Check sheet for the drawn part. Datum: minimum x, y, z corner. Units: mm. Give positions to 0.01 mm unless a question says otherwise; leave off trailing zeros. Write each loop counter-clockwise with the first axis right and the second up, starting at its lowest first coordinate (ties: lowest second). Pieces come first, ordered by that corner, then holes. Notation, with made-up numbers: M 25.5,80 L 47.5,80 A15 ccw 47.5,94 Z; hole C -25,2 d7. An arc over 180 degrees is marked long. Write item = value, one per line.
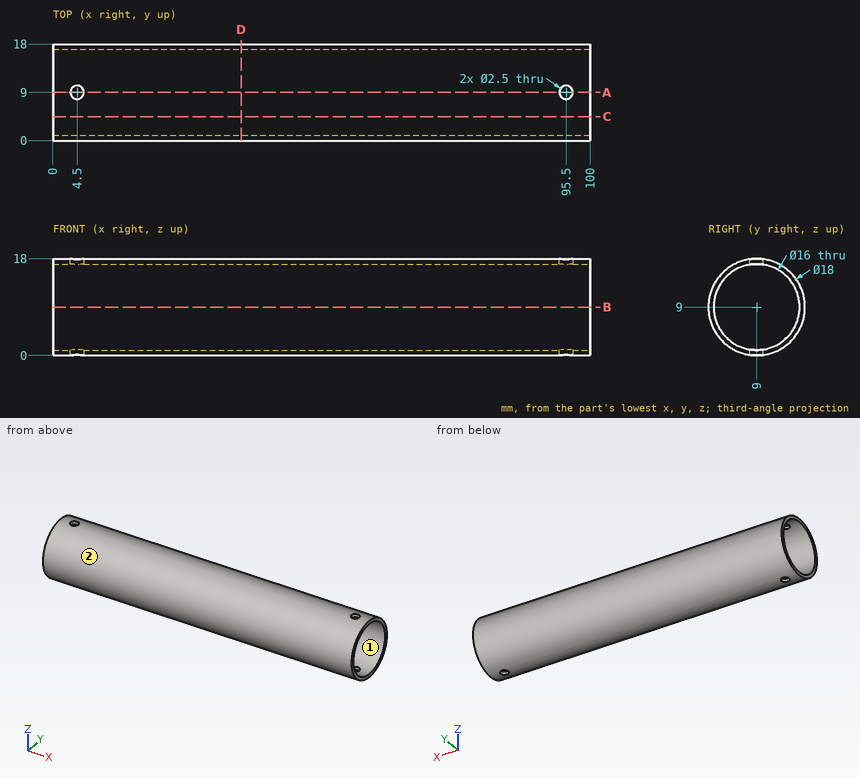
1) Cross-section at D-D on x = 35. Record the boundary of the cut face in (y, z), plus the area to 3 significant figures.
From the geometry:
outline = C 9,9 d18; hole C 9,9 d16
area = 53.4 mm^2
2) Cross-section at B-B on z = 9. Record the boundary of the cut face in (x, y).
From the geometry:
outline = M 0,0 L 100,0 L 100,1 L 0,1 Z; M 0,17 L 100,17 L 100,18 L 0,18 Z
3) Depth check by flat-ended pin: P1, Ø3, axis at x = 82.5, z = 3.5, coming from the +Y side; P2, Ø5, axis at x = 52, z = 5, coming from the -Y side; P3, Ø1.5, axis at x = 44.5, z = 8, coming from the +Y side. Enter the tip coordinate at first touch or a pass-through.
From the geometry:
P1 = 17.06
P2 = 0.13
P3 = 18
4) Cross-section at A-A on y = 9. Record the boundary of the cut face in (x, z), plus the area to 3 significant figures.
From the geometry:
outline = M 0,0 L 3.25,0 L 3.25,1 L 0,1 Z; M 0,17 L 3.25,17 L 3.25,18 L 0,18 Z; M 5.75,0 L 94.25,0 L 94.25,1 L 5.75,1 Z; M 5.75,17 L 94.25,17 L 94.25,18 L 5.75,18 Z; M 96.75,0 L 100,0 L 100,1 L 96.75,1 Z; M 96.75,17 L 100,17 L 100,18 L 96.75,18 Z
area = 190 mm^2
5) Draft check along Z on the marked faces 1 and 2. Enter one of: +Z half, -Z half, draft (parallel to the pull), parting line (faces both ways), or undercut.
From the geometry:
face_1 = undercut
face_2 = parting line
6) Cross-section at C-C on y = 4.5. Record the boundary of the cut face in (x, z), plus the area to 3 significant figures.
From the geometry:
outline = M 0,1.21 L 100,1.21 L 100,2.39 L 0,2.39 Z; M 0,15.61 L 100,15.61 L 100,16.79 L 0,16.79 Z
area = 236 mm^2
7) Material ranges on probe 1 along Z at (x, y) = (59, 2.75); probe 2 along Z at (x, y) = (94, 2); probe 3 along Y at (x, z) = (55, 5.75), recorded low to high. Write a range as from..to.
From the geometry:
probe_1 = 2.52..4.01, 13.99..15.48
probe_2 = 3.34..5.13, 12.87..14.66
probe_3 = 0.61..1.69, 16.31..17.39
